For this review, take the finished solid that the model builds, in its own axes (mm). A direction names the side the tool comes from. Coordinates: 2 decimals unless noted, no trailing zeros. Order: outer loops, then holes, each group sorted by start corner. A loop starts at its lowest first (then second) coordinate and runs counter-clockwise, first axis right, second up.
from build123d import *

# Parameters (mm, degrees)
F0_R            = 9
F0_R_2          = 4
F1_DEPTH        = 3
F2_R            = 4
F3_DEPTH        = 1
F4_R            = 0.5
F6_DEPTH        = 9.001
F6_COPIES_COUNT = 7
F10_R           = 0.5


# Not quite as in the source:
# - a pattern or mirror of a feature is missing from the dataset's text; its kind, count and spacing are read off the source's solid


with BuildPart() as f1:
    # F0 (on Top) → F1 (new body)
    with BuildSketch(Plane.XY):
        Circle(F0_R)
        Circle(F0_R_2, mode=Mode.SUBTRACT)
    extrude(amount=F1_DEPTH)

    # F2 (on face) → F3 (join)
    with BuildSketch(Plane(origin=(0, 0, 0), x_dir=(1, 0, 0), z_dir=(0, 0, -1))):
        Circle(F2_R)
    extrude(amount=-F3_DEPTH)

    # F4
    f4_edges = [f1.edges().sort_by_distance(p)[0] for p in [
        (-9, 0, 0),
        (-9, 0, 3),
    ]]
    fillet(f4_edges, radius=F4_R)

    # F5 (on Right) → F6 (cut, through all)
    with BuildSketch(Plane.YZ):
        Polygon((-0.2886751346, 0), (0.2886751346, 0), (0, 0.5), align=None)
    f6 = extrude(amount=-F6_DEPTH, mode=Mode.SUBTRACT)

    # F6_copies: F6 ×7 about axis
    f6_copies_axis = Axis((0, 0, 0), (0, 0, 1))
    for i in range(1, F6_COPIES_COUNT):
        add(f6.rotate(f6_copies_axis, i * 360 / F6_COPIES_COUNT), mode=Mode.SUBTRACT)

    # F7 (on Right) → F9 (revolve, cut)
    with BuildSketch(Plane.YZ):
        Polygon((4.5, 0.5), (4.2113248654, 0), (4.7886751346, 0), align=None)
    revolve(axis=Axis((0, 0, 0.5049179308), (0, 0, 1)), mode=Mode.SUBTRACT)

    # F10
    f10_edges = [f1.edges().sort_by_distance(p)[0] for p in [
        (-4, 0, 3),
    ]]
    fillet(f10_edges, radius=F10_R)


solid = f1.part
1. Machinability: for faces 3 (the face through (-0.867, -3.905, 1.74)), 4 (the face through (2, -2, 0)), which of the approach directions +Z, -Z, +X, -X, +Y, -Y give a long, thin tool a straight path to every point of the face, cutting with its end or side? Answer none if there is none.
Answer below:
face 3: +Z
face 4: -Z, +X, -X, +Y, -Y
2. Take a section at A-A, the plane z = 1.35. Give the boundary of the cut face in (x, y), plus the area to 3 significant figures.
Answer below:
outline: circle Ø18 at (0, 0); hole circle Ø8 at (0, 0)
area: 204 mm2
3. Clearance check with flat-ended pins moving along their axes: pin 1 Ø4 at (x, y) = (0.5, -0.5) entering from +Z; pin 2 Ø1 at (x, z) = (-6, 2.5) entering from +Y; pin 3 Ø1.5 at (x, y) = (-3, -2) entering from -Z. State where each tip first meets the part, or that it passes through.
Answer below:
pin 1: stops at z = 1
pin 2: stops at y = 7.12
pin 3: stops at z = 0
4. Take a section at B-B, the plane z = 2.75. Give the boundary of the cut face in (x, y).
Answer below:
outline: circle Ø17.87 at (0, 0); hole circle Ø8.13 at (0, 0)
5. To check wall thickness, follow L1, parallel to Y at x = 0, z = 1.6; L2, parallel to X at y = -2.5, z = 1.6. State the ranges of each line that lie inside material, in increasing order.
Answer below:
L1: y = -9 to -4, 4 to 9
L2: x = -8.65 to -3.12, 3.12 to 8.65
6. The part is to be moulded in two halves that separate along Y. For faces 1 (the face through (3, 0, 0)), 2 (the face through (0.35, 2.19, 0.25)), say which applies: +Y half, -Y half, draft (parallel to the pull), parting line (faces both ways), or undercut.
Answer below:
face 1: draft
face 2: undercut
